Source: CAD feature listing. Evaluate the final solid. Frame: model axes, mm. Face numbers are marked on the shaded views. A direction names the side the tool comes from. Give positions to 0.01 mm unless a question says otherwise; leave off trailing zeros. Write each loop counter-clockwise with the first axis right and the second up, starting at its lowest first coordinate (ties: lowest second). Pieces come first, ordered by that corner, then holes. Notation, with made-up numbers: (-20, 54) -> (24, 54) arc R20 ccw to (24, 86) -> close; hole circle Ø2 at (36, -18.5). An arc over 180 degrees is marked (long way). Use a Markdown table: item, result. Add a question column.
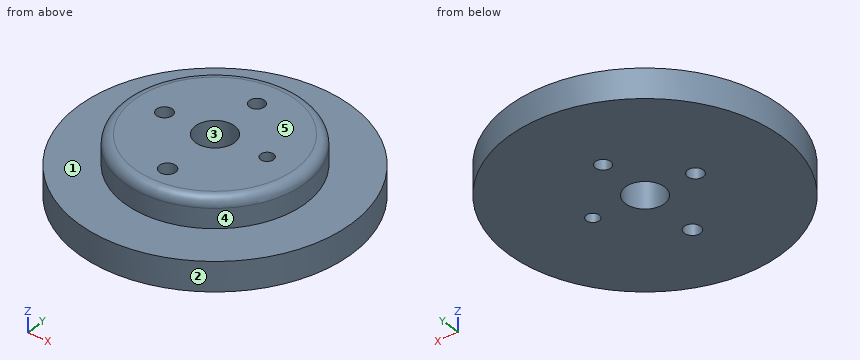
```python
from build123d import *

# Parameters (mm, degrees)
F0_R     = 14
F1_DEPTH = 3
F2_R     = 9.262684
F3_DEPTH = 3
F4_R     = 2
F5_DEPTH = 30
F6_R     = 0.780538
F6_R_2   = 0.67232
F6_R_3   = 0.833775
F6_R_4   = 0.807745
F7_DEPTH = 25.4
F8_R     = 1


with BuildPart() as f1:
    # F0 (on Top) → F1 (new body)
    with BuildSketch(Plane.XY):
        Circle(F0_R)
    extrude(amount=F1_DEPTH)

    # F2 (on face) → F3 (join)
    with BuildSketch(Plane.XY.offset(3)):
        Circle(F2_R)
    extrude(amount=F3_DEPTH)

    # F4 (on face) → F5 (cut)
    with BuildSketch(Plane.XY.offset(6)):
        Circle(F4_R)
    extrude(amount=-F5_DEPTH, mode=Mode.SUBTRACT)

    # F6 (on face) → F7 (cut)
    with BuildSketch(Plane.XY.offset(6)):
        with Locations((0, 5.578444)):
            Circle(F6_R)
        with Locations((5.356538, 0)):
            Circle(F6_R_2)
        with Locations((0, -6.308428)):
            Circle(F6_R_3)
        with Locations((-5.185302, 0)):
            Circle(F6_R_4)
    extrude(amount=-F7_DEPTH, mode=Mode.SUBTRACT)

    # F8
    f8_edges = [f1.edges().sort_by_distance(p)[0] for p in [
        (-9.262684, 0, 6),
    ]]
    fillet(f8_edges, radius=F8_R)


solid = f1.part
```
(1) Cut plane B-B on x = 0. Return the cut outline in (y, z).
(2) Mould query, pull axis Y, two halves, no side actions, for the marked faces 3, 4 and 5. Classes: +Y half, -Y half, draft (parallel to the pull), parting line (faces both ways), or undercut.
(3) Cut plane D-D on z = 2. Return the cut outline in (x, y), then the cut area to 3 significant figures.
(4) Access query for the marked faces 1 and 2. Directions: +Z, -Z, +X, -X, +Y, -Y. A direction counts if a zero-diameter tool reaches every point of the face in a straight line with its end or side. Return the directions, or none.
(5) Cut plane C-C on z = 4.05. Return the cut outline in (x, y).
(6) Material intervals for L1, parallel to Y at x = 0, z = 2.1; L2, parallel to Y at x = 0, z = 4.45; L3, parallel to Z at x = -8.5, y = 6.75, sorted ascending.
(7) First-contact query: pin 1 Ø6.5 at (x, y) = (0, 0) entering from +Z; pin 2 Ø1.5 at (x, z) = (-2.5, 4.5) entering from +Y. Flat tips, straight axial feed; report the tip coordinate or a pass-through.
(8) Cut plane A-A on y = 0. Return the cut outline in (x, z).
Output:
| question | item | result |
|---|---|---|
| 1 | outline | (-14, 0) -> (-7.14, 0) -> (-7.14, 6) -> (-8.26, 6) arc R1 ccw to (-9.26, 5) -> (-9.26, 3) -> (-14, 3) -> close; (-5.47, 0) -> (-2, 0) -> (-2, 6) -> (-5.47, 6) -> close; (2, 0) -> (4.8, 0) -> (4.8, 6) -> (2, 6) -> close; (6.36, 0) -> (14, 0) -> (14, 3) -> (9.26, 3) -> (9.26, 5) arc R1 ccw to (8.26, 6) -> (6.36, 6) -> close |
| 2 | face 3 | undercut |
| 2 | face 4 | parting line |
| 2 | face 5 | draft |
| 3 | outline | circle Ø28 at (0, 0); hole circle Ø1.62 at (-5.19, 0); hole circle Ø4 at (0, 0); hole circle Ø1.67 at (0, -6.31); hole circle Ø1.56 at (0, 5.58); hole circle Ø1.34 at (5.36, 0) |
| 3 | area | 596 mm^2 |
| 4 | face 1 | +Z |
| 4 | face 2 | +Z, -Z |
| 5 | outline | circle Ø18.53 at (0, 0); hole circle Ø1.62 at (-5.19, 0); hole circle Ø4 at (0, 0); hole circle Ø1.67 at (0, -6.31); hole circle Ø1.56 at (0, 5.58); hole circle Ø1.34 at (5.36, 0) |
| 6 | L1 | -14 to -7.14, -5.47 to -2, 2 to 4.8, 6.36 to 14 |
| 6 | L2 | -9.26 to -7.14, -5.47 to -2, 2 to 4.8, 6.36 to 9.26 |
| 6 | L3 | 0 to 3 |
| 7 | pin 1 | z = 6 |
| 7 | pin 2 | y = 9.1 |
| 8 | outline | (-14, 0) -> (-5.99, 0) -> (-5.99, 6) -> (-8.26, 6) arc R1 ccw to (-9.26, 5) -> (-9.26, 3) -> (-14, 3) -> close; (-4.38, 0) -> (-2, 0) -> (-2, 6) -> (-4.38, 6) -> close; (2, 0) -> (4.68, 0) -> (4.68, 6) -> (2, 6) -> close; (6.03, 0) -> (14, 0) -> (14, 3) -> (9.26, 3) -> (9.26, 5) arc R1 ccw to (8.26, 6) -> (6.03, 6) -> close |
